Geometry check sheet. Reference: the model listing, model coordinates, mm. Round coordinates to 2 decimals unless told otherwise and drop trailing zeros. Write each loop counter-clockwise with the first axis right and the second up, starting at its lowest first coordinate (ties: lowest second). Pieces come first, ordered by that corner, then holes. Notation, with made-up numbers: M -1.75,31.5 L 57.25,31.5 A16 ccw 57.25,37.5 Z; hole C 11,32.25 d7. An arc over 180 degrees is marked long. One line per item, written item: value. Start each with the question number.
1. Scan lines: probe 1 along Z at (x, y) = (68.5, 0); probe 2 along X at (y, z) = (5.25, -3.25); probe 3 along Y at (x, z) = (12.5, 0.25). Record each from-to range of solid material in increasing order. Write a range as [from, to].
2. Section check D-D (x = 48). Record the boundary of the cut face in (y, z).
3. Section check B-B (x = 69.5). Record the boundary of the cut face in (y, z).
4. Section check A-A (y = 0). Record the boundary of the cut face in (x, z).
5. Release check for a two-part mould opening along Y. For faces 1 (the flat face through (66.2, 0, 0)), 2 (the flat face through (0, 0, 0)), 3 (the cylindrical face through (33.56, -1.38, -6.2)) record: pulls with the +Y half, pulls with the -Y half, needs draft (parallel to the pull), parting line crosses it, or undercut.
6. Depth check by flat-ended pin: P1, Ø4, axis at x = 36.5, z = -4.5, coming from the -Y side. Enter the tip coordinate at first touch or a pass-through.
from build123d import *

# Parameters (mm, degrees)
F0_R     = 6
F1_DEPTH = 76.2
F2_SIZE  = 0.762
F4_D     = 5
F4_DEPTH = 16
F4_TIP   = 1.5021515476
F6_R     = 6.35
F7_DEPTH = 66.2


with BuildPart() as f1:
    # F0 (on Right) → F1 (new body)
    with BuildSketch(Plane.YZ):
        Circle(F0_R)
    extrude(amount=F1_DEPTH)

    # F2
    f2_edges = [f1.edges().sort_by_distance(p)[0] for p in [
        (76.2, -6, 0),
    ]]
    chamfer(f2_edges, length=F2_SIZE)

    # F4
    with Locations(Plane.YZ.offset(76.2)):
        with Locations((0, 0)):
            Hole(F4_D / 2, depth=F4_DEPTH)
            with Locations((0, 0, -(F4_DEPTH + F4_TIP / 2))):  # 118° drill point
                Cone(0, F4_D / 2, F4_TIP, mode=Mode.SUBTRACT)

    # F6 (on offset) → F7 (join, through all)
    with BuildSketch(Plane.YZ.offset(66.2)):
        Circle(F6_R)
    extrude(amount=-F7_DEPTH)


solid = f1.part
Result sheet:
1. probe 1: z = [-6, -2.5], [2.5, 6]
1. probe 2: x = [0, 66.2]
1. probe 3: y = [-6.35, 6.35]
2. outline: C 0,0 d12.7
3. outline: C 0,0 d12; hole C 0,0 d5
4. outline: M 0,-6.35 L 66.2,-6.35 L 66.2,-6 L 75.44,-6 L 76.2,-5.24 L 76.2,-2.5 L 66.2,-2.5 L 66.2,2.5 L 76.2,2.5 L 76.2,5.24 L 75.44,6 L 66.2,6 L 66.2,6.35 L 0,6.35 Z
5. face 1: undercut
5. face 2: needs draft
5. face 3: parting line crosses it
6. P1: stops at y = -5.84
